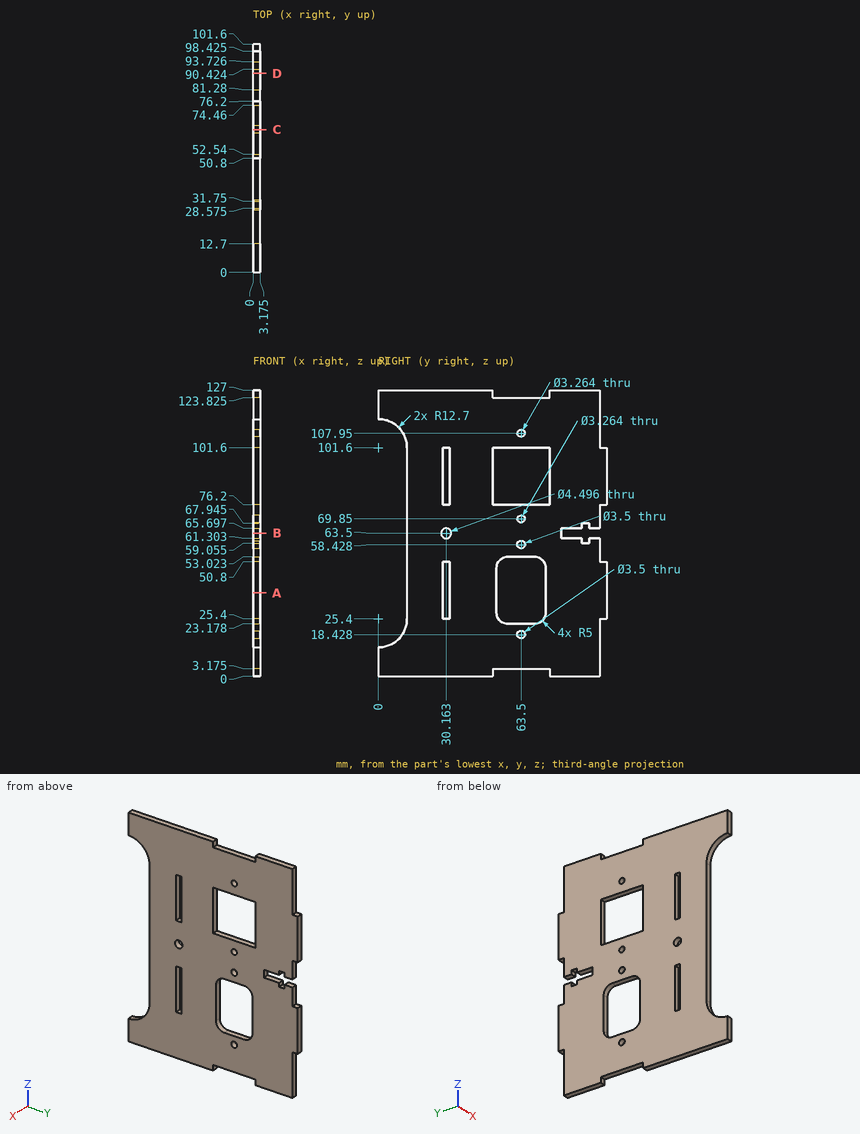
Part print with two shaded views. Sizes in mm from the minimum x, y, z corner. Coordinates: 2 decimals unless noted, no trailing zeros. Order: outer loops, then holes, each group sorted by start corner. A loop starts at its lowest first (then second) coordinate and runs counter-clockwise, first axis right, second up. Notation, with made-up numbers: (-28.5, 88.25) - (-0.5, 88.25) arc R6 cw to (-0.5, 93.25) - close; hole circle Ø2 at (31.5, -31). An arc over 180 degrees is marked (long way). Write item = value, one per line. Start each with the question number.
1) Wall check: line 1 along Z through (x, y) = (2.9, 30); line 2 along Y through (x, z) = (2.45, 66) (1 decimal); line 3 along Z through (x, y) = (0.2, 56) (1 decimal). Give the ranges that are in metal, low to high. Write a range as from..to.
2) Saw through at B-B on z = 63.5. Write the cut outline in (x, y) (1 decimal).
3) Saw through at D-D on y = 88.5. Write the cut outline in (x, z) (1 decimal).
4) Saw through at A-A on z = 37. Count the separate pieces of the cut face and the enclosed holes in it.
5) Saw through at C-C on y = 63.5. Write the cut outline in (x, z) (1 decimal).
6) Flat gauge pins, fed straight in: pin 1 Ø12 at (y, z) = (88.5, 18.5) entering from -X; pin 2 Ø1.5 at (x, z) = (2, 104.5) entering from +Y (1 decimal); pin 3 Ø1 at (x, y) = (1, 59.5) entering from +Z (1 decimal). Where does each tip first touch, or does it go through?
From the geometry:
q1.line_1 = 0..25.4, 50.8..61.26, 65.74..76.2, 101.6..127
q1.line_2 = 12.7..90.4, 93.7..98.4
q1.line_3 = 3.2..23.4, 52.8..76.2, 101.6..123.8
q2.outline = (0, 12.7) - (3.2, 12.7) - (3.2, 27.9) - (0, 27.9) - close; (0, 32.4) - (3.2, 32.4) - (3.2, 81.3) - (0, 81.3) - close
q3.outline = (0, 0) - (3.2, 0) - (3.2, 61.3) - (0, 61.3) - close; (0, 65.7) - (3.2, 65.7) - (3.2, 127) - (0, 127) - close
q4.separate_pieces = 3
q4.enclosed_holes = 0
q5.outline = (0, 3.2) - (3.2, 3.2) - (3.2, 16.7) - (0, 16.7) - close; (0, 20.2) - (3.2, 20.2) - (3.2, 23.2) - (0, 23.2) - close; (0, 53) - (3.2, 53) - (3.2, 56.7) - (0, 56.7) - close; (0, 60.2) - (3.2, 60.2) - (3.2, 68.2) - (0, 68.2) - close; (0, 71.5) - (3.2, 71.5) - (3.2, 76.2) - (0, 76.2) - close; (0, 101.6) - (3.2, 101.6) - (3.2, 106.3) - (0, 106.3) - close; (0, 109.6) - (3.2, 109.6) - (3.2, 123.8) - (0, 123.8) - close
q6.pin_1 = 0
q6.pin_2 = 98.4
q6.pin_3 = 123.8
